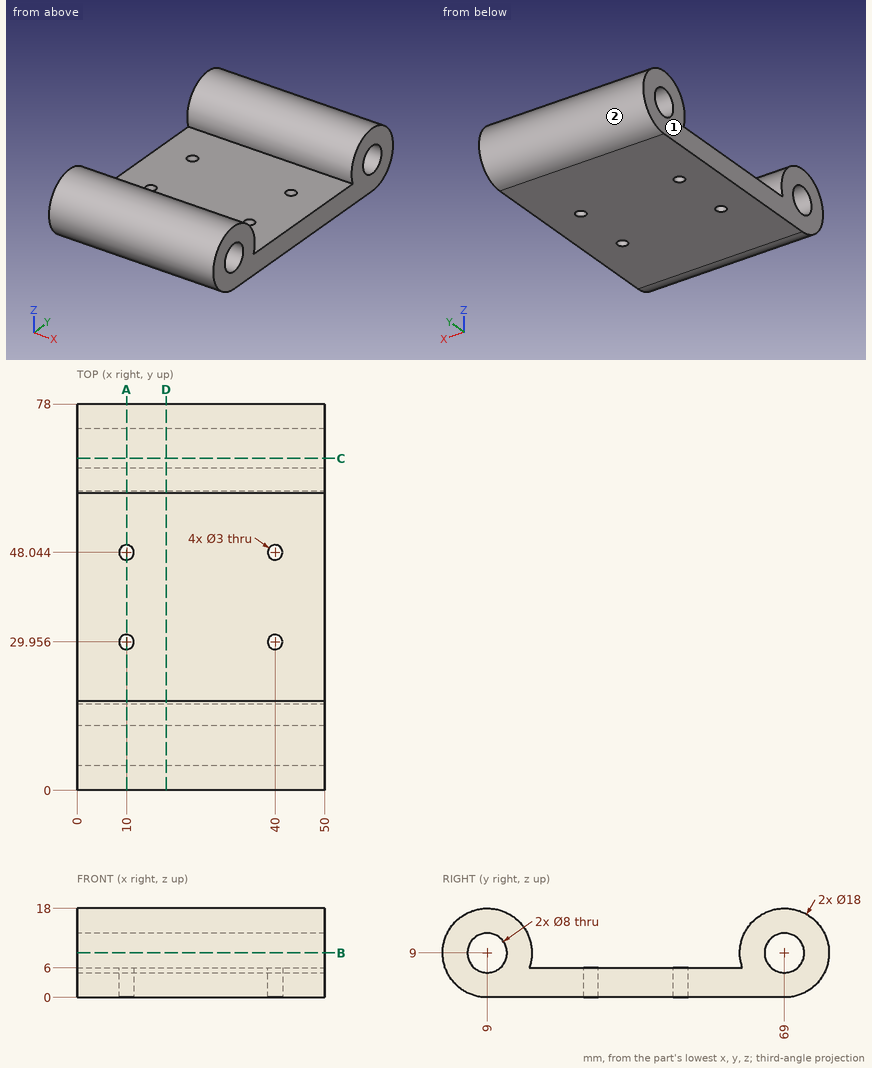
Check sheet for the drawn part. Datum: minimum x, y, z corner. Units: mm. Round coordinates to 2 decimals unless told otherwise and drop trailing zeros. Loops run counter-clockwise (first coordinate to the right, second up) from the corner with the lowest first, then second, coordinate; pieces in that order, holes last. Notation, with made-up numbers: (78, 51.5) - (117, 51.5) arc R23 cw to (117, 71.5) - close; hole circle Ø5 at (6, 35.25). An arc over 180 degrees is marked (long way). Write item = value, one per line. Start each with the question number.
1. Mould release check, pull along Y, two halves, no side actions. Record for the marked faces 1 and 2: released by +Y, released by -Y, zero draft, split by the parting line, or undercut.
2. Thickness scan on line 1 (Y direction, x = 29, z = 9); line 2 (Y direction, x = 40, z = 2.25) (1 decimal); line 3 (Y direction, x = 45.5, z = 6.5) (1 decimal). Record the ranges inside material, lowest first.
3. Section check B-B on z = 9. Enter the section's corners in (x, y).
4. Section check D-D on x = 18. Enter the section's corners in (y, z) (1 decimal).
5. Section check A-A on x = 10. Enter the section's corners in (y, z) (1 decimal).
6. Depth check by flat-ended pin: pin 1 (5 mm diameter, centred on x = 28.5, z = 14, fed in from +Y) (1 decimal); pin 2 (5 mm diameter, centred on x = 19, z = 2.5, fed in from +Y); pin 3 (1 mm diameter, centred on x = 26.5, z = 10, fed in from +Y); pin 4 (1.8 mm diameter, centred on x = 10, y = 29.96, fed in from +Z). Enter the tip coordinate at first touch or a pass-through.
7. Section check C-C on y = 67. Enter the section's corners in (x, z) (1 decimal).
Working result:
q1.face_1 = zero draft
q1.face_2 = undercut
q2.line_1 = 0 to 5, 13 to 18, 60 to 65, 73 to 78
q2.line_2 = 3 to 28.5, 31.5 to 46.5, 49.5 to 75
q2.line_3 = 0.4 to 5.9, 12.1 to 17.6, 60.4 to 65.9, 72.1 to 77.6
q3.outline = (0, 0) - (50, 0) - (50, 5) - (0, 5) - close; (0, 13) - (50, 13) - (50, 18) - (0, 18) - close; (0, 60) - (50, 60) - (50, 65) - (0, 65) - close; (0, 73) - (50, 73) - (50, 78) - (0, 78) - close
q4.outline = (9, 0) - (69, 0) arc R9 ccw (long way) to (60.5, 6) - (17.5, 6) arc R9 ccw (long way) to start; hole circle Ø8 at (9, 9); hole circle Ø8 at (69, 9)
q5.outline = (9, 0) - (28.5, 0) - (28.5, 6) - (17.5, 6) arc R9 ccw (long way) to start; (31.5, 0) - (46.5, 0) - (46.5, 6) - (31.5, 6) - close; (49.5, 0) - (69, 0) arc R9 ccw (long way) to (60.5, 6) - (49.5, 6) - close; hole circle Ø8 at (9, 9); hole circle Ø8 at (69, 9)
q6.pin_1 = 77.6
q6.pin_2 = 77.06
q6.pin_3 = 77.99
q6.pin_4 = through
q7.outline = (0, 0) - (50, 0) - (50, 5.5) - (0, 5.5) - close; (0, 12.5) - (50, 12.5) - (50, 17.8) - (0, 17.8) - close
